The listing builds one solid part. Answer for the finished solid, in the listing's coordinates (mm). A direction names the side the tool comes from. Give positions to 0.01 mm unless a question says otherwise; leave off trailing zeros. Write each loop counter-clockwise with the first axis right and the second up, starting at its lowest first coordinate (ties: lowest second). Pieces come first, ordered by that corner, then holes. Notation, with made-up numbers: (53, -0.75) -> (57, -0.75) arc R37 cw to (57, 37.25) -> close; hole circle Ø7 at (42.5, 62.25). An arc over 180 degrees is marked (long way). Put each result on its own line as item: value. Start each with the question number.
1) A cutting plane is placed at C-C (y = 35). Write down the section's boundary in (x, z), then the cut area to 3 significant figures.
2) A cutting plane is placed at D-D (z = -28). Write down the section's boundary in (x, y).
3) A flat-ended cylindrical pin translates along its axis: pin 1 Ø4 at (x, z) = (-48.5, -35) entering from +Y. Find the tip coordinate at first contact, or state that the pin passes through.
4) A cutting plane is placed at B-B (x = -53.5). Write down the section's boundary in (y, z).
5) For a pull along Y with two mould halves and no side action, classify faces 4 (the flat face through (-105, 46, -1)), 5 (the flat face through (-105, 48, -1)), 6 (the cylindrical face through (95.73, 46.99, -95.38)) as released by +Y, released by -Y, zero draft, split by the parting line, or undercut.
6) Find the intervals of material crossed by line 1 along Z through (x, y) = (12, 31); line 2 along X through (y, z) = (47.5, 16.5), in increasing order. Write a range as from..to.
7) For faces 1 (the cylindrical face through (-100.979, 24.65, -101.445)), 2 (the cylindrical face through (99.58, 23.692, 100.015)), 3 (the cylindrical face through (95.38, 46.99, 95.73)), determine the directions among +Z, -Z, +X, -X, +Y, -Y from which every point of the face is accessible in a straight line to the end or side of a thin tool.
from build123d import *

# Parameters (mm, degrees)
BOSS_EXTRUDE1_DEPTH = 50
SHELL1_T            = -2
CUT_EXTRUDE2_DEPTH  = 5
CUT_EXTRUDE4_DEPTH  = 5
BOSS_EXTRUDE3_START = 44
BOSS_EXTRUDE3_DEPTH = 2
CUT_EXTRUDE6_REACH  = 254.198
CUT_EXTRUDE6_START  = -1.2
CUT_EXTRUDE7_REACH  = 254.198
CUT_EXTRUDE7_START  = -1.2


with BuildPart() as part:
    # Sketch1 → Boss-Extrude1 (new body)
    with BuildSketch(Plane(origin=(0, 0, 0), x_dir=(1, 0, 0), z_dir=(0, 1, 0))):
        with BuildLine():
            Line((-80, -110), (80, -110))
            ThreePointArc((80, -110), (101.213203436, -101.213203436), (110, -80))
            Line((110, -80), (110, 80))
            ThreePointArc((110, 80), (101.213203436, 101.213203436), (80, 110))
            Line((80, 110), (-80, 110))
            ThreePointArc((-80, 110), (-101.213203436, 101.213203436), (-110, 80))
            Line((-110, 80), (-110, -80))
            ThreePointArc((-110, -80), (-101.213203436, -101.213203436), (-80, -110))
        make_face()
    extrude(amount=BOSS_EXTRUDE1_DEPTH)

    # Shell1
    shell1_openings = [part.faces().sort_by_distance(p)[0] for p in [
        (0, 50, 0),
    ]]
    offset(amount=SHELL1_T, openings=shell1_openings, kind=Kind.INTERSECTION)

    # Sketch5 → Cut-Extrude2 (cut)
    with BuildSketch(Plane(origin=(110, 0, 0), x_dir=(0, 0, -1), z_dir=(1, 0, 0))):
        with BuildLine():
            Line((-10.7, 16.8), (10.7, 16.8))
            ThreePointArc((10.7, 16.8), (13.9, 20), (10.7, 23.2))
            Line((10.7, 23.2), (-10.7, 23.2))
            ThreePointArc((-10.7, 23.2), (-13.9, 20), (-10.7, 16.8))
        make_face()
    extrude(amount=-CUT_EXTRUDE2_DEPTH, mode=Mode.SUBTRACT)

    # Sketch7 → Cut-Extrude4 (cut)
    with BuildSketch(Plane.XY.offset(110)):
        with BuildLine():
            Line((-10.7, 16.8), (10.7, 16.8))
            ThreePointArc((10.7, 16.8), (13.9, 20), (10.7, 23.2))
            Line((10.7, 23.2), (-10.7, 23.2))
            ThreePointArc((-10.7, 23.2), (-13.9, 20), (-10.7, 16.8))
        make_face()
    extrude(amount=-CUT_EXTRUDE4_DEPTH, mode=Mode.SUBTRACT)

    # Sketch8 → Boss-Extrude3 (add)
    with BuildSketch(Plane(origin=(0, 2, 0), x_dir=(1, 0, 0), z_dir=(0, 1, 0)).offset(BOSS_EXTRUDE3_START)):
        with BuildLine():
            Line((80, 108), (-80, 108))
            ThreePointArc((-80, 108), (-99.798989873, 99.798989873), (-108, 80))
            Line((-108, 80), (-108, -80))
            ThreePointArc((-108, -80), (-99.798989873, -99.798989873), (-80, -108))
            Line((-80, -108), (80, -108))
            ThreePointArc((80, -108), (99.798989873, -99.798989873), (108, -80))
            Line((108, -80), (108, 80))
            ThreePointArc((108, 80), (99.798989873, 99.798989873), (80, 108))
        make_face()
        with BuildLine():
            Line((-102, 80), (-102, -80))
            ThreePointArc((-102, -80), (-95.556349186, -95.556349186), (-80, -102))
            Line((-80, -102), (80, -102))
            ThreePointArc((80, -102), (95.556349186, -95.556349186), (102, -80))
            Line((102, -80), (102, 80))
            ThreePointArc((102, 80), (95.556349186, 95.556349186), (80, 102))
            Line((80, 102), (-80, 102))
            ThreePointArc((-80, 102), (-95.556349186, 95.556349186), (-102, 80))
        make_face(mode=Mode.SUBTRACT)
    extrude(amount=BOSS_EXTRUDE3_DEPTH)

    # Sketch5<5> → Cut-Extrude6 (cut, up to next)
    with BuildSketch(Plane(origin=(110, 0, 0), x_dir=(0, 0, -1), z_dir=(1, 0, 0)).offset(CUT_EXTRUDE6_START), mode=Mode.PRIVATE) as cut_extrude6_sk1:
        with BuildLine():
            Line((-10.7, 24.2), (10.7, 24.2))
            ThreePointArc((10.7, 24.2), (14.9, 20), (10.7, 15.8))
            Line((10.7, 15.8), (-10.7, 15.8))
            ThreePointArc((-10.7, 15.8), (-14.9, 20), (-10.7, 24.2))
        make_face()
        with BuildLine():
            Line((-10.7, 23.2), (10.7, 23.2))
            ThreePointArc((10.7, 23.2), (13.9, 20), (10.7, 16.8))
            Line((10.7, 16.8), (-10.7, 16.8))
            ThreePointArc((-10.7, 16.8), (-13.9, 20), (-10.7, 23.2))
        make_face(mode=Mode.SUBTRACT)
    cut_extrude6_tool1 = extrude(cut_extrude6_sk1.sketch, amount=-CUT_EXTRUDE6_REACH, mode=Mode.PRIVATE) & part.part
    add(cut_extrude6_tool1.solids().sort_by_distance((108.8, 20, 14.590387))[0], mode=Mode.SUBTRACT)

    # Sketch7<3> → Cut-Extrude7 (cut, up to next)
    with BuildSketch(Plane.XY.offset(110).offset(CUT_EXTRUDE7_START), mode=Mode.PRIVATE) as cut_extrude7_sk1:
        with BuildLine():
            Line((-10.7, 24.2), (10.7, 24.2))
            ThreePointArc((10.7, 24.2), (14.9, 20), (10.7, 15.8))
            Line((10.7, 15.8), (-10.7, 15.8))
            ThreePointArc((-10.7, 15.8), (-14.9, 20), (-10.7, 24.2))
        make_face()
        with BuildLine():
            Line((-10.7, 23.2), (10.7, 23.2))
            ThreePointArc((10.7, 23.2), (13.9, 20), (10.7, 16.8))
            Line((10.7, 16.8), (-10.7, 16.8))
            ThreePointArc((-10.7, 16.8), (-13.9, 20), (-10.7, 23.2))
        make_face(mode=Mode.SUBTRACT)
    cut_extrude7_tool1 = extrude(cut_extrude7_sk1.sketch, amount=-CUT_EXTRUDE7_REACH, mode=Mode.PRIVATE) & part.part
    add(cut_extrude7_tool1.solids().sort_by_distance((0, 23.890387, 108.8))[0], mode=Mode.SUBTRACT)


solid = part.part
Reply:
1. outline: (-110, -80) arc R30 ccw to (-80, -110) -> (80, -110) arc R30 ccw to (110, -80) -> (110, 80) arc R30 ccw to (80, 110) -> (-80, 110) arc R30 ccw to (-110, 80) -> close; hole (-108, -80) arc R28 ccw to (-80, -108) -> (80, -108) arc R28 ccw to (108, -80) -> (108, 80) arc R28 ccw to (80, 108) -> (-80, 108) arc R28 ccw to (-108, 80) -> close
1. area: 1,640 mm2
2. outline: (-110, 0) -> (110, 0) -> (110, 50) -> (108, 50) -> (108, 48) -> (102, 48) -> (102, 46) -> (108, 46) -> (108, 2) -> (-108, 2) -> (-108, 46) -> (-102, 46) -> (-102, 48) -> (-108, 48) -> (-108, 50) -> (-110, 50) -> close
3. pin 1: stops at y = 2
4. outline: (0, -110) -> (50, -110) -> (50, -108) -> (48, -108) -> (48, -102) -> (46, -102) -> (46, -108) -> (2, -108) -> (2, 108) -> (46, 108) -> (46, 102) -> (48, 102) -> (48, 108) -> (50, 108) -> (50, 110) -> (0, 110) -> close
5. face 4: undercut
5. face 5: released by +Y
5. face 6: zero draft
6. line 1: z = -110..-108, 108..110
6. line 2: x = -110..-102, 102..110
7. face 1: -Z, -X, +Y, -Y
7. face 2: none
7. face 3: +Y
